```python
from build123d import *

# Parameters (mm, degrees)
BOSS_EXTRUDE2_DEPTH    = 50
CUT_EXTRUDE5_OUTLINE_W = 6.3
CUT_EXTRUDE5_OUTLINE_H = 5.3
CUT_EXTRUDE5_DEPTH     = 10
FILLET2_R              = 0.5
SKETCH18_W             = 15
SKETCH18_H             = 15
BOSS_EXTRUDE3_DEPTH    = 15
SKETCH20_R             = 2.5
CUT_EXTRUDE6_DEPTH     = 4.9
SKETCH27_R             = 2.5
CUT_EXTRUDE11_DEPTH    = 4.9
SKETCH30_R             = 2.5
CUT_EXTRUDE12_DEPTH    = 4.9
CHAMFER1_SIZE          = 1
FILLET3_R              = 0.5
SKETCH31_W             = 50
SKETCH31_H             = 30
CUT_EXTRUDE13_DEPTH    = 74.484692283
FILLET4_R              = 0.25


# Read off the part's stored shape, not the designer's step: Cut-Extrude5
with BuildPart() as part:
    # Sketch3 → Boss-Extrude2 (new body)
    with BuildSketch(Plane(origin=(0, 0, 0), x_dir=(1, 0, 0), z_dir=(0, 1, 0))):
        Polygon((5, 44.7), (10.3, 44.7), (10.3, 46.7), (15, 43.7), (5, 43.7), (5, 6.3), (15, 6.3), (10.3, 3.3), (10.3, 5.3), (5, 5.3), (5, 0), (0, 0), (0, 50), (5, 50), align=None)
    extrude(amount=BOSS_EXTRUDE2_DEPTH)

    # Cut-Extrude5 outline → Cut-Extrude5 (cut)
    with BuildSketch(Plane(origin=(5, 0, 0), x_dir=(0, 0, -1), z_dir=(1, 0, 0))):
        with Locations((3.15, 2.65)):
            Rectangle(CUT_EXTRUDE5_OUTLINE_W, CUT_EXTRUDE5_OUTLINE_H)
        with Locations((3.15, 47.35)):
            Rectangle(CUT_EXTRUDE5_OUTLINE_W, CUT_EXTRUDE5_OUTLINE_H)
        with Locations((46.85, 2.65)):
            Rectangle(CUT_EXTRUDE5_OUTLINE_W, CUT_EXTRUDE5_OUTLINE_H)
        with Locations((46.85, 47.35)):
            Rectangle(CUT_EXTRUDE5_OUTLINE_W, CUT_EXTRUDE5_OUTLINE_H)
    extrude(amount=CUT_EXTRUDE5_DEPTH, mode=Mode.SUBTRACT)

    # Fillet2
    fillet2_edges = [part.edges().sort_by_distance(p)[0] for p in [
        (10.3, 25, -46.7),
        (10.3, 25, -3.3),
    ]]
    fillet(fillet2_edges, radius=FILLET2_R)

    # Sketch18 → Boss-Extrude3 (add)
    with BuildSketch(Plane.ZY):
        with Locations((-25, 25)):
            Rectangle(SKETCH18_W, SKETCH18_H)
    extrude(amount=BOSS_EXTRUDE3_DEPTH)

    # Sketch20 → Cut-Extrude6 (cut)
    with BuildSketch(Plane(origin=(0, 32.5, 0), x_dir=(1, 0, 0), z_dir=(0, 1, 0))):
        with Locations(Location((-7.5, 25, 0), (0, 0, 270))):
            Circle(SKETCH20_R)
    extrude(amount=-CUT_EXTRUDE6_DEPTH, mode=Mode.SUBTRACT)

    # Sketch27 → Cut-Extrude11 (cut)
    with BuildSketch(Plane.XY.offset(-17.5)):
        with Locations((-7.5, 25)):
            Circle(SKETCH27_R)
    extrude(amount=-CUT_EXTRUDE11_DEPTH, mode=Mode.SUBTRACT)

    # Sketch30 → Cut-Extrude12 (cut)
    with BuildSketch(Plane.ZY.offset(15)):
        with Locations((-25, 25)):
            Circle(SKETCH30_R)
    extrude(amount=-CUT_EXTRUDE12_DEPTH, mode=Mode.SUBTRACT)

    # Chamfer1
    chamfer1_edges = [part.edges().sort_by_distance(p)[0] for p in [
        (-7.5, 17.5, -17.5),
        (-7.5, 32.5, -17.5),
        (-7.5, 32.5, -32.5),
        (-7.5, 17.5, -32.5),
        (-15, 25, -17.5),
        (-15, 32.5, -25),
        (-15, 25, -32.5),
        (-15, 17.5, -25),
    ]]
    chamfer(chamfer1_edges, length=CHAMFER1_SIZE)

    # Fillet3
    fillet3_edges = [part.edges().sort_by_distance(p)[0] for p in [
        (-7.5, 32.5, -27.5),
        (-10, 25, -17.5),
        (-15, 25, -27.5),
    ]]
    fillet(fillet3_edges, radius=FILLET3_R)

    # Sketch31 → Cut-Extrude13 (cut, through all)
    with BuildSketch(Plane(origin=(5, 0, 0), x_dir=(0, 0, -1), z_dir=(1, 0, 0))):
        with Locations((25, 25)):
            Rectangle(SKETCH31_W, SKETCH31_H)
    extrude(amount=CUT_EXTRUDE13_DEPTH, mode=Mode.SUBTRACT)

    # Fillet4
    fillet4_edges = [part.edges().sort_by_distance(p)[0] for p in [
        (15, 7.65, -43.7),
        (15, 7.65, -6.3),
        (15, 42.35, -43.7),
        (15, 42.35, -6.3),
    ]]
    fillet(fillet4_edges, radius=FILLET4_R)


solid = part.part
```
For this review, take the finished solid that the model builds, in its own axes (mm). A direction names the side the tool comes from. Round coordinates to 2 decimals unless told otherwise and drop trailing zeros. Loops run counter-clockwise (first coordinate to the right, second up) from the corner with the lowest first, then second, coordinate; pieces in that order, holes last.
(1) We need section D-D (x = -2). Give the boundary of the cut face in (y, z).
Returned:
outline: (17.5, -31.5) - (18.5, -32.5) - (31.5, -32.5) - (32.5, -31.5) - (32.5, -18.5) - (31.5, -17.5) - (18.5, -17.5) - (17.5, -18.5) - close
(2) Wall thickness on line 1 along X through (y, z) = (12.5, -28); line 2 along Y through (x, z) = (-11.15, -25); line 3 along X through (y, z) = (26.5, -28): over which ranges is each line inside the solid? List them lowest first.
Returned:
line 1: x = 0 to 5
line 2: y = 17.5 to 22.5, 27.5 to 32.5
line 3: x = -15 to 5
(3) We need section A-A (x = -11.25). Give the boundary of the cut face in (y, z), plus the area to 3 significant figures.
Returned:
outline: (17.5, -31.5) - (18.5, -32.5) - (31.5, -32.5) - (32.5, -31.5) - (32.5, -18.5) - (31.5, -17.5) - (18.5, -17.5) - (17.5, -18.5) - close; hole circle Ø5 at (25, -25)
area: 203 mm2
(4) We need section B-B (z = -25). Give the boundary of the cut face in (x, y).
Returned:
outline: (-15, 18.5) - (-14, 17.5) - (0, 17.5) - (0, 0) - (5, 0) - (5, 50) - (0, 50) - (0, 32.5) - (-4.5, 32.5) arc R0.5 ccw to (-5, 32) - (-5, 27.6) - (-10, 27.6) - (-10, 32) arc R0.5 ccw to (-10.5, 32.5) - (-14, 32.5) - (-15, 31.5) - (-15, 28) arc R0.5 ccw to (-14.5, 27.5) - (-10.1, 27.5) - (-10.1, 22.5) - (-14.5, 22.5) arc R0.5 ccw to (-15, 22) - close
(5) Tool access review of faces 1 (the flat face through (-7, 17.5, -25)), 2 (the flat face through (8, 8, -5.3)), 3 (the flat face through (11, 44.7, -6)), 4 (the cylindrical face through (-12.33, 27.48, -25.33)): name each direction out of +Z, -Z, +X, -X, +Y, -Y from which nothing blocks a thin tool from reaching the whole face with its end or side.
Returned:
face 1: +Z, -Z, -X, -Y
face 2: +Z, +Y, -Y
face 3: +Z, -Z, +X, +Y
face 4: -X
(6) We need section C-C (y = 25). Give the boundary of the cut face in (x, z), plus the area to 3 significant figures.
Returned:
outline: (-15, -31.5) - (-14, -32.5) - (0, -32.5) - (0, -50) - (5, -50) - (5, 0) - (0, 0) - (0, -17.5) - (-4.5, -17.5) arc R0.5 ccw to (-5, -18) - (-5, -22.4) - (-10, -22.4) - (-10, -18) arc R0.5 ccw to (-10.5, -17.5) - (-14, -17.5) - (-15, -18.5) - (-15, -22) arc R0.5 ccw to (-14.5, -22.5) - (-10.1, -22.5) - (-10.1, -27.5) - (-14.5, -27.5) arc R0.5 ccw to (-15, -28) - close
area: 425 mm2
(7) Mouldability with a two-part tool opening along Z and no side actions: class faces 5 (the flat face through (10, 5.3, -44)), 6 (the flat face through (8, 42, -5.3)), 7 (the flat face through (-10.1, 25, -25)), 8 (the flat face through (-7, 25, -32.5)) as released by +Z, released by -Z, zero draft, split by the parting line, or undercut.
Returned:
face 5: zero draft
face 6: released by +Z
face 7: undercut
face 8: released by -Z
(8) Clearance check with flat-ended pins moving along their axes: P1, Ø5, axis at x = 6.5, z = -13, coming from the -Y side; P2, Ø6, axis at x = -5, z = -36, coming from the +Y side; P3, Ø3, axis at x = 11.5, z = -5, coming from the -Y side; P4, Ø2, axis at y = 34.5, z = -5, coming from the -X side. State where each tip first meets the part, or that it passes through.
Returned:
P1: stops at y = 0
P2: passes through
P3: stops at y = 5.3
P4: stops at x = 0
